```python
from build123d import *

# Parameters (mm, degrees)
SKETCH1_W           = 105
SKETCH1_H           = 35
BOSS_EXTRUDE1_DEPTH = 5
CUT_EXTRUDE1_DEPTH  = 5
SKETCH3_R           = 2.5
BOSS_EXTRUDE2_DEPTH = 5
CUT_EXTRUDE3_START  = -3.5
SKETCH4_R           = 2.5
SKETCH4_R_2         = 1.5
CUT_EXTRUDE3_DEPTH  = 1.5
CUT_EXTRUDE4_DEPTH  = 5
SKETCH6_W           = 1
SKETCH6_H           = 5.473396058
SKETCH6_H_2         = 2.850644757
SKETCH6_H_3         = 4.642061194
SKETCH6_H_4         = 3.194118723
CUT_EXTRUDE5_DEPTH  = 10


with BuildPart() as part:
    # Sketch1 → Boss-Extrude1 (new body)
    with BuildSketch(Plane.XY):
        with Locations((7.7, 5.6)):
            Rectangle(SKETCH1_W, SKETCH1_H)
    extrude(amount=BOSS_EXTRUDE1_DEPTH)

    # Sketch2 → Cut-Extrude1 (cut)
    with BuildSketch(Plane.XY.offset(5)):
        with BuildLine():
            Line((-34.8, -3.4), (-24.8, -3.4))
            ThreePointArc((-24.8, -3.4), (-21.3, -6.9), (-24.8, -10.4))
            Line((-24.8, -10.4), (-34.8, -10.4))
            ThreePointArc((-34.8, -10.4), (-38.3, -6.9), (-34.8, -3.4))
        make_face()
    extrude(amount=-CUT_EXTRUDE1_DEPTH, mode=Mode.SUBTRACT)

    # Sketch3 → Boss-Extrude2 (add)
    with BuildSketch(Plane(origin=(0, 0, 0), x_dir=(-1, 0, 0), z_dir=(0, 0, -1))):
        with Locations(Location((8.8, -6.9, 0), (0, 0, 180))):
            Circle(SKETCH3_R)
    extrude(amount=BOSS_EXTRUDE2_DEPTH)

    # Sketch4 → Cut-Extrude3 (cut)
    with BuildSketch(Plane(origin=(0, 0, -5), x_dir=(-1, 0, 0), z_dir=(0, 0, -1)).offset(CUT_EXTRUDE3_START)):
        with Locations(Location((8.8, -6.9, 0), (0, 0, 180))):
            Circle(SKETCH4_R)
        with Locations((8.8, -6.9)):
            Circle(SKETCH4_R_2, mode=Mode.SUBTRACT)
    extrude(amount=CUT_EXTRUDE3_DEPTH, mode=Mode.SUBTRACT)

    # Sketch5 → Cut-Extrude4 (cut)
    with BuildSketch(Plane(origin=(0, 0, 0), x_dir=(-1, 0, 0), z_dir=(0, 0, -1))):
        Polygon((-41.2, 0.1), (-50.2, 0.1), (-50.2, 10.1), (-45.7, 10.1), (-52.7, 20.1), (-41.2, 20.1), align=None)
        Polygon((-20.2, 0.1), (-29.2, 0.1), (-29.2, 10.1), (-24.7, 10.1), (-31.7, 20.1), (-20.2, 20.1), align=None)
        Polygon((1.05, 0.1), (-7.95, 0.1), (-7.95, 10.1), (-3.45, 10.1), (-10.45, 20.1), (1.05, 20.1), align=None)
        Polygon((22.3, 0.1), (13.3, 0.1), (13.3, 10.1), (17.8, 10.1), (10.8, 20.1), (22.3, 20.1), align=None)
        Polygon((43.55, 0.1), (34.55, 0.1), (34.55, 10.1), (39.05, 10.1), (32.05, 20.1), (43.55, 20.1), align=None)
    extrude(amount=-CUT_EXTRUDE4_DEPTH, mode=Mode.SUBTRACT)

    # Sketch6 → Cut-Extrude5 (cut)
    with BuildSketch(Plane(origin=(0, 0, 0), x_dir=(-1, 0, 0), z_dir=(0, 0, -1))):
        with Locations((-46.2, 10.54511412)):
            Rectangle(SKETCH6_W, SKETCH6_H)
        with Locations((-25.2, 10.54511412)):
            Rectangle(SKETCH6_W, SKETCH6_H)
        with Locations((-3.95, 10.654861904)):
            Rectangle(SKETCH6_W, SKETCH6_H_2)
        with Locations((17.3, 10.960781552)):
            Rectangle(SKETCH6_W, SKETCH6_H_3)
        with Locations((38.55, 10.826598887)):
            Rectangle(SKETCH6_W, SKETCH6_H_4)
    extrude(amount=-CUT_EXTRUDE5_DEPTH, mode=Mode.SUBTRACT)


solid = part.part
```
Geometry check sheet. Reference: the model listing, model coordinates, mm. A direction names the side the tool comes from. Give positions to 0.01 mm unless a question says otherwise; leave off trailing zeros. Loops run counter-clockwise (first coordinate to the right, second up) from the corner with the lowest first, then second, coordinate; pieces in that order, holes last. Notation, with made-up numbers: (-37.5, -6) - (-33.5, -6) arc R9 ccw to (-33.5, 10) - close; hole circle Ø6 at (-15, 67). An arc over 180 degrees is marked (long way). Use CSV: the item, a comma, the result in double quotes. Start each with the question number.
Q1. Section check B-B, the plane y = -6.9. Record the cut outline in (x, z).
Q2. Scan lines: probe 1 along X at (y, z) = (19, 0.5); probe 2 along Y at (x, z) = (-36.5, 3); probe 3 along X at (y, z) = (19.5, 2). Record each from-to range of solid material in increasing order. Write a range as from..to.
Q3. Release check for a two-part mould opening along X. For faces 1 (the face through (7, -11.9, 2)), 2 (the face through (-15, 10.1, 2)), 3 (the face through (-9.13, -9.38, -3.99)) record: +X half, -X half, draft (parallel to the pull), parting line (faces both ways), or undercut.
Q4. Go/stop test with flat-tipped pins: pin 1 Ø1.5 at (x, y) = (2, -3.5) entering from -Z; pin 2 Ø6 at (x, z) = (47, -1) entering from -Y. Record where each tip stops, or that it passes through.
Q5. Access from +Z, -Z, +X, -X, +Y, -Y to the whole of each face (thin tool, end or side, straight path). Record for faces 4 (the face through (-43.55, 10, 2)), 5 (the face through (-10, -6, -2)), 6 (the face through (19, 6, 5)).
Q6. Section check D-D, the plane x = 49. Record the cut outline in (y, z).
Q7. Section check A-A, the plane y = 18. Record the cut outline in (x, z), and give its area (3 significant figures).
Q8. Section check C-C, the plane x = -23.5. Record the cut outline in (y, z), and give its area (3 significant figures).
Findings below:
1,outline,"(-44.8, 0) - (-38.3, 0) - (-38.3, 5) - (-44.8, 5) - close; (-21.3, 0) - (-11.3, 0) - (-11.3, -1.5) - (-10.3, -1.5) - (-10.3, -3) - (-11.3, -3) - (-11.3, -5) - (-6.3, -5) - (-6.3, -3) - (-7.3, -3) - (-7.3, -1.5) - (-6.3, -1.5) - (-6.3, 0) - (60.2, 0) - (60.2, 5) - (-21.3, 5) - close"
2,probe 1,"x = -44.8..-43.55, -32.82..-22.3, -11.57..-1.05, 9.68..20.2, 30.93..41.2, 51.93..60.2"
2,probe 2,"y = -11.9..-9.96, -3.84..0.1, 10.1..13.74, 20.1..23.1"
2,probe 3,"x = -44.8..-43.55, -32.47..-22.3, -11.22..-1.05, 10.03..20.2, 31.28..41.2, 52.28..60.2"
3,face 1,"draft"
3,face 2,"undercut"
3,face 3,"parting line"
4,pin 1,"stops at z = 0"
4,pin 2,"stops at y = -11.9"
5,face 4,"+Z, -Z"
5,face 5,"none"
5,face 6,"+Z, +X, -X, +Y, -Y"
6,outline,"(-11.9, 0) - (0.1, 0) - (0.1, 5) - (-11.9, 5) - close; (10.1, 0) - (14.81, 0) - (14.81, 5) - (10.1, 5) - close; (20.1, 0) - (23.1, 0) - (23.1, 5) - (20.1, 5) - close"
7,outline,"(-44.8, 0) - (-43.55, 0) - (-43.55, 5) - (-44.8, 5) - close; (-33.52, 0) - (-22.3, 0) - (-22.3, 5) - (-33.52, 5) - close; (-12.27, 0) - (-1.05, 0) - (-1.05, 5) - (-12.27, 5) - close; (8.98, 0) - (20.2, 0) - (20.2, 5) - (8.98, 5) - close; (30.23, 0) - (41.2, 0) - (41.2, 5) - (30.23, 5) - close; (51.23, 0) - (60.2, 0) - (60.2, 5) - (51.23, 5) - close"
7,area,"274 mm^2"
8,outline,"(-11.9, 0) - (-10.15, 0) - (-10.15, 5) - (-11.9, 5) - close; (-3.65, 0) - (23.1, 0) - (23.1, 5) - (-3.65, 5) - close"
8,area,"143 mm^2"
